from build123d import *

# Parameters (mm, degrees)
BOSS_EXTRUDE1_DEPTH = 4


with BuildPart() as part:
    # Sketch1 → Boss-Extrude1 (new body)
    with BuildSketch(Plane(origin=(0, 0, 0), x_dir=(1, 0, 0), z_dir=(0, 1, 0))):
        with BuildLine():
            Line((-287.599492609, 307.846688721), (-276.509158993, 96.230517076))
            add(Edge.make_bspline(
                [(-276.509158993, 96.230517076), (-265.498754924, -193.422418568), (-100.154473104, -360.089981136), (-97.455270859, -365.359331923)],
                knots=[0, 0, 0, 0, 1, 1, 1, 1], degree=3))
            Line((-97.455270859, -365.359331923), (-100.871017472, -299.24345381))
            add(Edge.make_bspline(
                [(-247.476970144, 99.184701956), (-209.870171036, -233.687963111), (-103.612719847, -283.411888875), (-100.871017472, -299.24345381)],
                knots=[0, 0, 0, 0, 1, 1, 1, 1], degree=3))
            Line((-247.476970144, 99.184701956), (-258.335189119, 309.358571318))
            Line((-258.335189119, 309.358571318), (-287.599492609, 307.846688721))
        make_face()
        with BuildLine():
            Line((-6.962227222, 322.345260258), (3.895991753, 112.171390896))
            add(Edge.make_bspline(
                [(3.895991753, 112.171390896), (0.792272957, -222.80450289), (-99.775370482, -283.213639779), (-100.871017472, -299.24345381)],
                knots=[0, 0, 0, 0, 1, 1, 1, 1], degree=3))
            Line((-100.871017472, -299.24345381), (-97.455270859, -365.359331923))
            add(Edge.make_bspline(
                [(33.078047071, 112.224730275), (51.975289253, -177.020747413), (-95.313450893, -359.839879259), (-97.455270859, -365.359331923)],
                knots=[0, 0, 0, 0, 1, 1, 1, 1], degree=3))
            Line((33.078047071, 112.224730275), (22.302076268, 323.857142855))
            Line((22.302076268, 323.857142855), (-6.962227222, 322.345260258))
        make_face()
    extrude(amount=BOSS_EXTRUDE1_DEPTH)


solid = part.part
Read the model definition and answer for the solid it produces. Units are mm, in the model's axes. Round coordinates to 2 decimals unless told otherwise and drop trailing zeros. Order: outer loops, then holes, each group sorted by start corner. A loop starts at its lowest first (then second) coordinate and runs counter-clockwise, first axis right, second up. Notation, with made-up numbers: (13.5, 37.5) - (48.5, 37.5) arc R18 ccw to (48.5, 65.5) - close; hole circle Ø1 at (-36, 40.25). An arc over 180 degrees is marked (long way). Use one line per item in the form item = value. Start each with the question number.
(1) Find the intervals of material crossed by line 1 along X through (y, z) = (2.4, 182); line 2 along X through (y, z) = (2, 194.5); line 3 along Z through (x, y) = (-57, 3), in increasing order. Write a range as from..to.
(2) The part is cut by section B-B (z = -243). Give the vertices of the cut face in (x, y), then the cut area to 3 significant figures.
(3) Flat-ended cylindrical pins translate along their axes: pin 1 Ø2 at (y, z) = (1.5, 164) entering from +X; pin 2 Ø2 at (x, y) = (-103, 1.5) entering from +Z. Find the tip coordinate at first contact, or state that the pin passes through.
(4) The part is cut by section A-A (z = -173). Give the vertices of the cut face in (x, y).
Checked values:
q1.line_1 = -213.01..-179.66, -37.12..-5.01
q1.line_2 = -207.39..-173.84, -41.66..-9.35
q1.line_3 = 229.85..300.72
q2.outline = (-284.2, 0) - (-254.91, 0) - (-254.91, 4) - (-284.2, 4) - close; (-2.86, 0) - (26.42, 0) - (26.42, 4) - (-2.86, 4) - close
q2.area = 234 mm^2
q3.pin_1 = 1.12
q3.pin_2 = 359.93
q4.outline = (-280.53, 0) - (-251.29, 0) - (-251.29, 4) - (-280.53, 4) - close; (0.75, 0) - (29.98, 0) - (29.98, 4) - (0.75, 4) - close
